Could you check a few things on this model? Use its own coordinates, in mm. A direction names the side the tool comes from. Round coordinates to 2 decimals unless told otherwise and drop trailing zeros. Loops run counter-clockwise (first coordinate to the right, second up) from the corner with the lowest first, then second, coordinate; pieces in that order, holes last. Notation, with made-up numbers: (-29, 28.5) -> (13, 28.5) arc R17 ccw to (13, 52.5) -> close; hole circle Ø2 at (68.25, 41). An arc over 180 degrees is marked (long way). Write each question's results on one line, items separated by ' | '.
from build123d import *

# Parameters (mm, degrees)
SKETCH2_W               = 43.3
SKETCH2_H               = 71.19
SKETCH2_W_2             = 31.3
SKETCH2_H_2             = 59.19
BOSS_EXTRUDE1_DEPTH     = 5
SKETCH3_W               = 8.89
SKETCH3_H               = 6
BOSS_EXTRUDE2_DEPTH     = 8.8
CUT_EXTRUDE1_DEPTH      = 76.678124977
CUT_EXTRUDE1_DEPTH_BACK = 76.678124977
SKETCH5_R               = 2.2479
SKETCH8_W               = 11.205
SKETCH8_H               = 59.19
BOSS_EXTRUDE4_DEPTH     = 5
SKETCH9_W               = 9
SKETCH9_H               = 71.19
SKETCH9_W_2             = 2.21
SKETCH9_H_2             = 59.19
CUT_EXTRUDE2_DEPTH      = 5
SKETCH10_W              = 0.42
SKETCH10_H              = 59.19
BOSS_EXTRUDE5_DEPTH     = 5
SKETCH11_W              = 0.42
SKETCH11_H              = 71.19
CUT_EXTRUDE3_DEPTH      = 5
SKETCH12_W              = 6.655
SKETCH12_H              = 10.668
BOSS_EXTRUDE6_DEPTH     = 5
SKETCH13_W              = 8.205
SKETCH13_H              = 6
CUT_EXTRUDE4_DEPTH      = 5
SKETCH14_W              = 2
SKETCH14_H              = 10.668
CUT_EXTRUDE5_DEPTH      = 5
SKETCH15_W              = 5
SKETCH15_H              = 12.7
BOSS_EXTRUDE7_DEPTH     = 4.62
SKETCH16_W              = 10.785
SKETCH16_H              = 10.668
BOSS_EXTRUDE8_DEPTH     = 5
SKETCH17_W              = 6
SKETCH17_H              = 3
CUT_EXTRUDE6_DEPTH      = 5
SKETCH18_R              = 1.47
CUT_EXTRUDE7_DEPTH      = 5
SKETCH23_R              = 1.47
CUT_EXTRUDE10_DEPTH     = 5
SKETCH25_W              = 6.445
SKETCH25_H              = 2.583619091
BOSS_EXTRUDE12_DEPTH    = 5
SKETCH26_W              = 15.24
SKETCH26_H              = 8.382
SKETCH26_W_2            = 19.675
SKETCH26_H_2            = 6.066644496
SKETCH26_W_3            = 2.21
CUT_EXTRUDE11_DEPTH     = 5


with BuildPart() as part:
    # Sketch2 → Boss-Extrude1 (new body)
    with BuildSketch(Plane.XY):
        Rectangle(SKETCH2_W, SKETCH2_H)
        Rectangle(SKETCH2_W_2, SKETCH2_H_2, mode=Mode.SUBTRACT)
    extrude(amount=BOSS_EXTRUDE1_DEPTH)

    # Sketch3 → Boss-Extrude2 (add)
    with BuildSketch(Plane.XY.offset(5)):
        with Locations((0, 32.595)):
            Rectangle(SKETCH3_W, SKETCH3_H)
        with Locations((0, -32.595)):
            Rectangle(SKETCH3_W, SKETCH3_H)
    extrude(amount=BOSS_EXTRUDE2_DEPTH)

    # Sketch5 → Cut-Extrude1 (cut, two sides: drawn at the far end of the back side and taken through both)
    with BuildSketch(Plane(origin=(0, 35.595, 0), x_dir=(1, 0, 0), z_dir=(0, 1, 0)).offset(-CUT_EXTRUDE1_DEPTH_BACK)):
        with BuildLine():
            Line((-4.445, -13.8), (-2.8e-08, -13.8))
            ThreePointArc((-2.8e-08, -13.8), (-3.127220221, -12.513973022), (-4.445, -9.4))
            Line((-4.445, -9.4), (-4.445, -13.8))
        make_face()
        with BuildLine():
            Line((4.445, -13.8), (4.445, -9.4))
            ThreePointArc((4.445, -9.4), (3.127220202, -12.513973041), (-2.8e-08, -13.8))
            Line((-2.8e-08, -13.8), (4.445, -13.8))
        make_face()
        with Locations(Location((0, -9.354769886, 0), (0, 0, 90))):
            Circle(SKETCH5_R)
    extrude(amount=CUT_EXTRUDE1_DEPTH + CUT_EXTRUDE1_DEPTH_BACK, mode=Mode.SUBTRACT)

    # Sketch8 → Boss-Extrude4 (add)
    with BuildSketch(Plane.XY.offset(5)):
        with Locations((10.0475, 0)):
            Rectangle(SKETCH8_W, SKETCH8_H)
    extrude(amount=-BOSS_EXTRUDE4_DEPTH)

    # Sketch9 → Cut-Extrude2 (cut)
    with BuildSketch(Plane.XY.offset(5)):
        with Locations((17.15, 0)):
            Rectangle(SKETCH9_W, SKETCH9_H)
        with Locations((5.55, 0)):
            Rectangle(SKETCH9_W_2, SKETCH9_H_2)
    extrude(amount=-CUT_EXTRUDE2_DEPTH, mode=Mode.SUBTRACT)

    # Sketch10 → Boss-Extrude5 (add)
    with BuildSketch(Plane.XY.offset(5)):
        with Locations((-15.44, 0)):
            Rectangle(SKETCH10_W, SKETCH10_H)
    extrude(amount=-BOSS_EXTRUDE5_DEPTH)

    # Sketch11 → Cut-Extrude3 (cut)
    with BuildSketch(Plane.XY.offset(5)):
        with Locations((-21.44, 0)):
            Rectangle(SKETCH11_W, SKETCH11_H)
    extrude(amount=-CUT_EXTRUDE3_DEPTH, mode=Mode.SUBTRACT)

    # Sketch12 → Boss-Extrude6 (add)
    with BuildSketch(Plane.XY.offset(5)):
        with Locations((3.3275, -24.261)):
            Rectangle(SKETCH12_W, SKETCH12_H)
    extrude(amount=-BOSS_EXTRUDE6_DEPTH)

    # Sketch13 → Cut-Extrude4 (cut)
    with BuildSketch(Plane.XY.offset(5)):
        with Locations((8.5475, -32.595)):
            Rectangle(SKETCH13_W, SKETCH13_H)
    extrude(amount=-CUT_EXTRUDE4_DEPTH, mode=Mode.SUBTRACT)

    # Sketch14 → Cut-Extrude5 (cut)
    with BuildSketch(Plane.XY.offset(5)):
        with Locations((1, -24.261)):
            Rectangle(SKETCH14_W, SKETCH14_H)
    extrude(amount=-CUT_EXTRUDE5_DEPTH, mode=Mode.SUBTRACT)

    # Sketch15 → Boss-Extrude7 (add)
    with BuildSketch(Plane.ZY.offset(21.23)):
        with Locations((2.5, -29.245)):
            Rectangle(SKETCH15_W, SKETCH15_H)
    extrude(amount=BOSS_EXTRUDE7_DEPTH)

    # Sketch16 → Boss-Extrude8 (add)
    with BuildSketch(Plane.XY.offset(5)):
        with Locations((-9.8375, -24.261)):
            Rectangle(SKETCH16_W, SKETCH16_H)
    extrude(amount=-BOSS_EXTRUDE8_DEPTH)

    # Sketch17 → Cut-Extrude6 (cut)
    with BuildSketch(Plane.XY.offset(5)):
        with Locations((-17.65, -29.095)):
            Rectangle(SKETCH17_W, SKETCH17_H)
        Polygon((-25.85, -30.595), (-25.85, -35.595), (-14.65, -35.595), (-14.65, -30.595), (-20.65, -30.595), align=None)
    extrude(amount=-CUT_EXTRUDE6_DEPTH, mode=Mode.SUBTRACT)

    # Sketch18 → Cut-Extrude7 (cut)
    with BuildSketch(Plane.XY.offset(5)):
        with Locations((-23.31, -27.625)):
            Circle(SKETCH18_R)
    extrude(amount=-CUT_EXTRUDE7_DEPTH, mode=Mode.SUBTRACT)

    # Sketch23 → Cut-Extrude10 (cut)
    with BuildSketch(Plane.XY.offset(5)):
        with Locations((-18.23, 24.405)):
            Circle(SKETCH23_R)
        with Locations((9.68, 24.405)):
            Circle(SKETCH23_R)
    extrude(amount=-CUT_EXTRUDE10_DEPTH, mode=Mode.SUBTRACT)

    # Sketch25 → Boss-Extrude12 (add)
    with BuildSketch(Plane.XY.offset(5)):
        Polygon((6.655, -27.011380909), (6.655, -8.796355504), (-15.23, -8.796355504), (-15.23, -18.927), (-4.445, -18.927), (-4.445, -27.011380909), (2, -27.011380909), align=None)
        with Locations((-1.2225, -28.303190455)):
            Rectangle(SKETCH25_W, SKETCH25_H)
    extrude(amount=-BOSS_EXTRUDE12_DEPTH)

    # Sketch26 → Cut-Extrude11 (cut)
    with BuildSketch(Plane.XY.offset(5)):
        with Locations((-3.175, -22.229)):
            Rectangle(SKETCH26_W, SKETCH26_H)
        with Locations((-5.3925, -11.829677752)):
            Rectangle(SKETCH26_W_2, SKETCH26_H_2)
        with Locations((5.55, -11.829677752)):
            Rectangle(SKETCH26_W_3, SKETCH26_H_2)
    extrude(amount=-CUT_EXTRUDE11_DEPTH, mode=Mode.SUBTRACT)


solid = part.part
1) I want a section at C-C, the plane x = -10. Write out the boundary of the cut face in (y, z) (3 decimals).
Model answer:
outline: (-35.595, 0) -> (-26.42, 0) -> (-26.42, 5) -> (-35.595, 5) -> close; (-18.038, 0) -> (-14.863, 0) -> (-14.863, 5) -> (-18.038, 5) -> close; (29.595, 0) -> (35.595, 0) -> (35.595, 5) -> (29.595, 5) -> close
2) I need wall thicknesses on line 1 (Y direction, x = -18.23, z = 3.65) (3 decimals); line 2 (Y direction, x = 3, z = 12.5) (3 decimals); line 3 (X direction, y = 21.5, z = 1) (3 decimals). Which ranges of each line are inside material? Lowest first, please.
Model answer:
line 1: y = -27.595 to 22.935, 25.875 to 35.595 | line 2: y = -35.595 to -29.595, 29.595 to 35.595 | line 3: x = -21.23 to -15.23, 6.655 to 12.65
3) I'm going to push flat-ended pins straight in: pin 1 (5 mm diameter, centred on y = -33, z = 4.5, fed in from +X) (3 decimals); pin 2 (2 mm diameter, centred on y = 33.5, z = 7, fed in from -X) (3 decimals); pin 3 (5.5 mm diameter, centred on x = 9, z = 3, fed in from -Y) (3 decimals). Where does each tip first touch, or does it pass through?
Model answer:
pin 1: stops at x = 4.445 | pin 2: stops at x = -4.445 | pin 3: stops at y = -29.595
4) For faces 1 (the flat face through (-18, -27.595, 3)), 2 (the flat face through (-3, -18.038, 3)), 3 (the flat face through (8, -29.595, 3)), 4 (the flat face through (4.445, 33, 7)), which set-ups out of +Z, -Z, +X, -X, +Y, -Y let a thin tool reach every point of the face, with its end or its side?
Model answer:
face 1: +Z, -Z, -Y | face 2: +Z, -Z | face 3: +Z, -Z, +X, -Y | face 4: +Z, +X, +Y, -Y
5) I want a section at A-A, the plane z = 5.75. Write out the boundary of the cut face in (x, y) (3 decimals), plus the area to 3 significant figures.
Model answer:
outline: (-4.445, -35.595) -> (4.445, -35.595) -> (4.445, -29.595) -> (-4.445, -29.595) -> close; (-4.445, 29.595) -> (4.445, 29.595) -> (4.445, 35.595) -> (-4.445, 35.595) -> close | area: 107 mm2
6) I want a section at D-D, the plane z = 10.75. Write out the boundary of the cut face in (x, y) (1 decimal), plus the area to 3 significant figures.
Model answer:
outline: (-4.2, -35.6) -> (-1.8, -35.6) -> (-1.8, -29.6) -> (-4.2, -29.6) -> close; (-4.2, 29.6) -> (-1.8, 29.6) -> (-1.8, 35.6) -> (-4.2, 35.6) -> close; (1.8, -35.6) -> (4.2, -35.6) -> (4.2, -29.6) -> (1.8, -29.6) -> close; (1.8, 29.6) -> (4.2, 29.6) -> (4.2, 35.6) -> (1.8, 35.6) -> close | area: 59.0 mm2
7) If we mould it in two halves opening along Y, with no side actions, what happens to faces 5 (the flat face through (-2, 29.595, 5)), 6 (the flat face through (4.445, -33, 5)), 7 (the cylindrical face through (-18.55, 22.97, 2.54)), 8 (the flat face through (-3, -35.595, 5))? For each: released by +Y, released by -Y, zero draft, split by the parting line, or undercut.
Model answer:
face 5: undercut | face 6: zero draft | face 7: undercut | face 8: released by -Y
8) I want a section at B-B, the plane x = -23.31. Write out the boundary of the cut face in (y, z) (3 decimals).
Model answer:
outline: (-30.595, 0) -> (-29.095, 0) -> (-29.095, 5) -> (-30.595, 5) -> close; (-26.155, 0) -> (-22.895, 0) -> (-22.895, 5) -> (-26.155, 5) -> close
